Input: part model. Units: mm. Frame: model coordinates. A direction names the side the tool comes from. Coordinates: 2 decimals unless noted, no trailing zeros. Order: outer loops, then holes, each group sorted by start corner. A loop starts at its lowest first (then second) coordinate and runs counter-clockwise, first axis right, second up. Notation, with made-up numbers: M 21,80.5 L 46,80.5 A21 ccw 46,92.5 Z; hole C 33,-40 d7. An arc over 180 degrees is marked long. Answer in a Markdown table with one row per item.
Autodesk Inventor part; units mm, degrees
ref_plane "YZ Plane" through (0, 0, 0) normal (1, 0, 0) x (0, 1, 0)
ref_plane "XZ Plane" through (0, 0, 0) normal (0, 1, 0) x (-1, 0, 0)
ref_plane "XY Plane" through (0, 0, 0) normal (0, 0, 1) x (1, 0, 0)
sketch "Esquisse1" plane through (0, 0, 0) normal (0, 0, 1) x (1, 0, 0)
  circle A0 centre (0, 0) radius 13
  dimension "d0" = 26
extrude "Extrusion1" add sketch "Esquisse1" along normal blind 110
sketch "Esquisse2" plane through (0, 0, 0) normal (0, 0, -1) x (-1, 0, 0)
  circle A0 centre (0, 0) radius 7
  circle A1 centre (0, 10) radius 1
  circle A2 centre (0, 0) radius 13
  circle A3 centre (-10, 0) radius 1
  circle A4 centre (0, -10) radius 1
  circle A5 centre (10, 0) radius 1
  dimension "d3" = 14
  dimension "d4" = 2
  dimension "d5" = 2
  dimension "d8" = 360
extrude "Extrusion2" cut sketch "Esquisse2" against normal blind 5 contours A1 | A3 | A4 | A5
sketch "Esquisse3" plane through (0, 0, 0) normal (0, 0, -1) x (-1, 0, 0)
  circle A0 centre (0, 0) radius 7
  dimension "d12" = 14
extrude "Extrusion3" add sketch "Esquisse3" along normal blind 2
sketch "Esquisse4" plane through (0, 0, -2) normal (0, 0, -1) x (-1, 0, 0)
  circle A0 centre (0, 0) radius 2.5
  dimension "d15" = 5
extrude "Extrusion4" add sketch "Esquisse4" along normal blind 14
properties part number "MoteurMaxon"
1) Cut plane A-A, the plane y = -5.5. Output: boundary loops of the cut face in (x, z), and give its area (3 significant figures).
Resolved:
| item | result |
|---|---|
| outline | M -11.78,0 L -4.33,0 L -4.33,-2 L 4.33,-2 L 4.33,0 L 11.78,0 L 11.78,110 L -11.78,110 Z |
| area | 2,610 mm2 |
2) Cut plane D-D, the plane z = 71. Output: boundary loops of the cut face in (x, y), and give its area (3 significant figures).
Resolved:
| item | result |
|---|---|
| outline | C 0,0 d26 |
| area | 531 mm2 |
3) Reachability of faces 1 (the face through (10, 0, 5)), 2 (the face through (-10.316, 7.91, 54.23)) from +Z, -Z, +X, -X, +Y, -Y: full face, straight path, thin tool, end or side. Return the list, or none.
Resolved:
| item | result |
|---|---|
| face 1 | -Z |
| face 2 | +Z, -Z |
4) Material intervals for probe 1 along Y at (x, z) = (0, 2.95); probe 2 along Z at (x, y) = (0.5, 2.75); probe 3 along Y at (x, z) = (10, 3.15), sorted ascending.
Resolved:
| item | result |
|---|---|
| probe 1 | y = -13 to -11, -9 to 9, 11 to 13 |
| probe 2 | z = -2 to 110 |
| probe 3 | y = -8.31 to -1, 1 to 8.31 |
5) Mould query, pull axis Y, two halves, no side actions, for faces 3 (the face through (0, 0, 110)), 4 (the face through (0.54, 2.44, -8.9)), 5 (the face through (10.8, -0.6, 2.5)). Classes: +Y half, -Y half, draft (parallel to the pull), parting line (faces both ways), or undercut.
Resolved:
| item | result |
|---|---|
| face 3 | draft |
| face 4 | parting line |
| face 5 | undercut |
6) Cut plane C-C, the plane z = -7.5. Output: boundary loops of the cut face in (x, y), and give its area (3 significant figures).
Resolved:
| item | result |
|---|---|
| outline | C 0,0 d5 |
| area | 19.6 mm2 |
7) Cut plane B-B, the plane x = -4.5. Output: boundary loops of the cut face in (y, z).
Resolved:
| item | result |
|---|---|
| outline | M -12.2,0 L -5.36,0 L -5.36,-2 L 5.36,-2 L 5.36,0 L 12.2,0 L 12.2,110 L -12.2,110 Z |
8) Contact query for flat-ended pins moving along their axis: pin 1 (0.6 mm diameter, centred on x = -10.5, y = 0, fed in from -Z); pin 2 (3 mm diameter, centred on x = 10, y = 0, fed in from -Z); pin 3 (8 mm diameter, centred on y = 9.5, z = 58.5, fed in from +X). Output: stop coordinate, or through.
Resolved:
| item | result |
|---|---|
| pin 1 | stops at z = 5 |
| pin 2 | stops at z = 0 |
| pin 3 | stops at x = 11.78 |
